CAD build for the part. Positions are in the model's coordinates, mm. Face numbers are marked on the shaded views. Coordinates: 2 decimals unless noted, no trailing zeros. Loops run counter-clockwise (first coordinate to the right, second up) from the corner with the lowest first, then second, coordinate; pieces in that order, holes last. Notation, with made-up numbers: (72.25, -27.5) -> (123.25, -27.5) arc R35 ccw to (123.25, 8.5) -> close; hole circle Ø1 at (-8.75, 35.5). An arc over 180 degrees is marked (long way). Return JSON: item names as keys, results as strings. Group by question number.
(1) Saw through at B-B on x = 22. Write the cut outline in (y, z), then the cut area to 3 significant figures.
(2) Saw through at A-A on x = 13.5. Write the cut outline in (y, z).
(3) Flat gauge pins, fed straight in: pin 1 Ø6 at (x, z) = (6, -21) entering from +Y; pin 2 Ø3 at (x, z) = (14.5, 18.5) entering from -Y; pin 3 Ø1.5 at (x, y) = (4.5, 12.5) entering from -Z; pin 4 Ø3 at (x, y) = (12, -9) entering from +Z. Where does each tip first touch, or does it go through?
(4) Saw through at C-C on x = 4. Write the cut outline in (y, z).
(5) Probe L1, parallel to Y at x = 6, z = 0; L2, parallel to X at y = -12, z = 11.5; L3, parallel to Z at x = 11, y = 0. List the from-to ranges inside material, lowest first.
(6) Mould opens along Z. For the marked faces 1, 2 and 3 say: pulls with the +Z half, pulls with the -Z half, needs draft (parallel to the pull), parting line crosses it, or undercut.
```python
from build123d import *

# Parameters (mm, degrees)
F3_D     = 16
F3_DEPTH = 15
F3_TIP   = 4.8068849522
F4_SIZE  = 2
F5_SIZE  = 1


with BuildPart() as f1:
    # F0 (on Front) → F1 (revolve)
    with BuildSketch(Plane.XZ):
        Polygon((0, 14), (0, 0), (25, 0), (25, 27.5), (10, 27.5), (10, 14), align=None)
    revolve(axis=Axis((12.5, 0, 0), (-1, 0, 0)))

    # F3
    with Locations(Plane(origin=(0, 0, 0), x_dir=(0, -1, 0), z_dir=(-1, 0, 0))):
        with Locations((0, 0)):
            Hole(F3_D / 2, depth=F3_DEPTH)
            with Locations((0, 0, -(F3_DEPTH + F3_TIP / 2))):  # 118° drill point
                Cone(0, F3_D / 2, F3_TIP, mode=Mode.SUBTRACT)

    # F4
    f4_edges = [f1.edges().sort_by_distance(p)[0] for p in [
        (25, 0, -27.5),
        (10, 0, -27.5),
        (17.5, 0, 27.5),
    ]]
    chamfer(f4_edges, length=F4_SIZE)

    # F5
    f5_edges = [f1.edges().sort_by_distance(p)[0] for p in [
        (0, 0, -14),
    ]]
    chamfer(f5_edges, length=F5_SIZE)


solid = f1.part
```
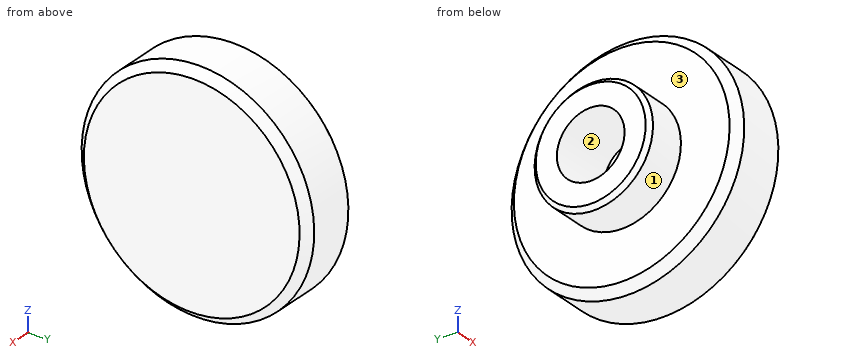
Geometry results:
{
 "1": {"outline": "circle Ø55 at (0, 0)", "area": "2,380 mm²"},
 "2": {"outline": "circle Ø55 at (0, 0); hole circle Ø16 at (0, 0)"},
 "3": {"pin 1": "through", "pin 2": "y = -21.62", "pin 3": "z = -7.61", "pin 4": "z = 26.46"},
 "4": {"outline": "circle Ø28 at (0, 0); hole circle Ø16 at (0, 0)"},
 "5": {"L1": "-14 to -8, 8 to 14", "L2": "10 to 25", "L3": "-26.5 to -8, 8 to 26.5"},
 "6": {"face 1": "parting line crosses it", "face 2": "undercut", "face 3": "needs draft"}
}
